CAD build for the part. Positions are in the model's coordinates, mm. A direction names the side the tool comes from. Round coordinates to 2 decimals unless told otherwise and drop trailing zeros. Loops run counter-clockwise (first coordinate to the right, second up) from the corner with the lowest first, then second, coordinate; pieces in that order, holes last. Notation, with made-up numbers: M 48,76 L 82,76 A25 cw 82,109 Z; hole C 1.25,6.25 d11. An arc over 180 degrees is marked long. Use one line per item in the form item = value.
from build123d import *

# Parameters (mm, degrees)
F0_W     = 50
F0_H     = 20
F1_DEPTH = 5
F3_DEPTH = 25
F4_W     = 0.4809010029
F4_H     = 3
F4_W_2   = 0.5
F4_H_2   = 2
F4_H_3   = 1
F5_DEPTH = 25
F7_DEPTH = 25


with BuildPart() as f1:
    # F0 (on Top) → F1 (new body)
    with BuildSketch(Plane.XY):
        with Locations((25, 10)):
            Rectangle(F0_W, F0_H)
    extrude(amount=F1_DEPTH)

    # F2 (on face) → F3 (cut)
    with BuildSketch(Plane.XZ):
        Polygon((0, 5), (0, 0), (42.5, 5), align=None)
    extrude(amount=-F3_DEPTH, mode=Mode.SUBTRACT)

    # F4 (on face) → F5 (cut)
    with BuildSketch(Plane.XZ):
        Polygon((42.5, 5), (34, 4), (42, 4), (42.5, 4), align=None)
        Polygon((34, 4), (25.5, 3), (33.5, 3), (34, 3), align=None)
        Polygon((25.5, 3), (17, 2), (25.0037251041, 2), (25, 2.0037817754), (25.5, 2), align=None)
        Polygon((17, 2), (8.5, 1), (16.5, 1), (17, 1), align=None)
        Polygon((17, 1), (16.5, 1), (16.75, 0.75), align=None)
        Polygon((25, 2.0037817754), (25.0037251041, 2), (25.5, 2), align=None)
        Polygon((25.5, 2), (25.0037251041, 2), (25.2481091664, 1.7518980383), align=None)
        Polygon((34, 3), (33.5, 3), (33.75, 2.75), align=None)
        Polygon((42.5, 4), (42, 4), (42.25, 3.75), align=None)
        Polygon((17, 0), (16.75, 0.25), (16.5, 0), align=None)
        with Locations((42.2595494986, 1.5)):
            Rectangle(F4_W, F4_H)
        with Locations((33.75, 1)):
            Rectangle(F4_W_2, F4_H_2)
        with Locations((25.25, 0.5)):
            Rectangle(F4_W_2, F4_H_3)
    extrude(amount=-F5_DEPTH, mode=Mode.SUBTRACT)

    # F6 (on face) → F7 (cut)
    with BuildSketch(Plane.XZ):
        Polygon((8.5, 0), (8.5, 1), (0, 0), align=None)
    extrude(amount=-F7_DEPTH, mode=Mode.SUBTRACT)


solid = f1.part
1. Tool access for faces 1 (the face through (42.5, 10, 1)), 2 (the face through (33.6, 20, 2.5)), 3 (the face through (12, 10, 1)): list every direction of +Z, -Z, +X, -X, +Y, -Y with a clear straight run to the whole face (end or side of a thin tool).
Completed:
face_1 = -Z, +Y, -Y
face_2 = +Z, -Z, +X, -X, +Y
face_3 = +Z, -X, +Y, -Y
2. Probe line 1 along X through (y, z) = (9.75, 0.65); line 2 along X through (y, z) = (1, 1.3); line 3 along X through (y, z) = (17.25, 2.2). List the from-to ranges inside material, lowest first. Write a range as from..to.
Completed:
line_1 = 8.5..25, 25.5..33.5, 34..42.02, 42.5..50
line_2 = 17..33.5, 34..42.02, 42.5..50
line_3 = 25.5..42.02, 42.5..50
3. Cut at A-A on z = 4.5. Write the cut outline in (x, y).
Completed:
outline = M 42.5,0 L 50,0 L 50,20 L 42.5,20 Z
4. Cut at B-B on x = 38. Write the cut outline in (y, z), and give its area (3 significant figures).
Completed:
outline = M 0,0 L 20,0 L 20,4 L 0,4 Z
area = 80.0 mm2
5. Drop flat-ended pins along their axis: P1, Ø0.8, axis at y = 6, z = 2.5, coming from the -X side; P2, Ø2.5, axis at x = 20, y = 7.5, coming from the +Z side; P3, Ø6, axis at x = 33, y = 9.5, coming from the +Z side; P4, Ø2, axis at x = 18, z = 4, coming from the -Y side. Give the stop position or say it passes through.
Completed:
P1 = 25.5
P2 = 2
P3 = 4
P4 = through
